Verification items for the finished model (mm, model axes). A direction names the side the tool comes from. Give positions to 0.01 mm unless a question says otherwise; leave off trailing zeros. Write each loop counter-clockwise with the first axis right and the second up, starting at its lowest first coordinate (ties: lowest second). Pieces come first, ordered by that corner, then holes. Notation, with made-up numbers: M 63.25,9.5 L 72.25,9.5 A30 ccw 72.25,40.5 Z; hole C 59,-30.5 d1. An arc over 180 degrees is marked long. Write item = value, one per line.
from build123d import *

# Parameters (mm, degrees)
F0_W     = 76.2
F0_H     = 76.2
F1_DEPTH = 25.4
F2_W     = 12.7
F2_H     = 76.2
F6_DEPTH = 25.4
F4_W     = 76.2
F4_H     = 12.7
F7_DEPTH = 25.4
F5_W     = 76.2
F5_H     = 12.7
F8_DEPTH = 25.4
F3_W     = 12.7
F3_H     = 76.2
F9_DEPTH = 25.4


with BuildPart() as f1:
    # F0 (on Top) → F1 (new body)
    with BuildSketch(Plane.XY):
        with Locations((0.213519, -0.247781)):
            Rectangle(F0_W, F0_H)
    extrude(amount=F1_DEPTH)

    # F2 (on Top) → F6 (join)
    with BuildSketch(Plane.XY):
        with Locations((0.173656, 75.769984)):
            Rectangle(F2_W, F2_H)
    extrude(amount=F6_DEPTH)

    # F4 (on Top) → F7 (join)
    with BuildSketch(Plane.XY):
        with Locations((-75.986146, -0.193442)):
            Rectangle(F4_W, F4_H)
    extrude(amount=F7_DEPTH)

    # F5 (on Top) → F8 (join)
    with BuildSketch(Plane.XY):
        with Locations((76.36796, -0.207913)):
            Rectangle(F5_W, F5_H)
    extrude(amount=F8_DEPTH)

    # F3 (on Top) → F9 (join)
    with BuildSketch(Plane.XY):
        with Locations((0.085362, -76.094228)):
            Rectangle(F3_W, F3_H)
    extrude(amount=F9_DEPTH)


solid = f1.part
1) Material ranges on probe 1 along Y at (x, z) = (-19.5, 1.5); probe 2 along X at (y, z) = (-29.5, 14); probe 3 along Y at (x, z) = (41, 16), recorded low to high. Write a range as from..to.
From the geometry:
probe_1 = -38.35..37.85
probe_2 = -37.89..38.31
probe_3 = -6.56..6.14
2) Cross-section at B-B on y = 53. Record the boundary of the cut face in (x, z), plus the area to 3 significant figures.
From the geometry:
outline = M -6.18,0 L 6.52,0 L 6.52,25.4 L -6.18,25.4 Z
area = 323 mm^2
3) Cross-section at A-A on z = 14. Record the boundary of the cut face in (x, y), plus the area to 3 significant figures.
From the geometry:
outline = M -114.09,-6.54 L -37.89,-6.54 L -37.89,-38.35 L -6.26,-38.35 L -6.26,-114.19 L 6.44,-114.19 L 6.44,-38.35 L 38.31,-38.35 L 38.31,-6.56 L 114.47,-6.56 L 114.47,6.14 L 38.31,6.14 L 38.31,37.85 L 6.52,37.85 L 6.52,113.87 L -6.18,113.87 L -6.18,37.85 L -37.89,37.85 L -37.89,6.16 L -114.09,6.16 Z
area = 9,670 mm^2
4) Depth check by flat-ended pin: P1, Ø7.5, axis at x = 23, z = 9, coming from the -Y side; P2, Ø12.5, axis at x = -58, z = 11, coming from the -Y side; P3, Ø12.5, axis at x = 77.5, z = 16, coming from the -Y side. Enter the tip coordinate at first touch or a pass-through.
From the geometry:
P1 = -38.35
P2 = -6.54
P3 = -6.56
5) Cross-section at C-C on x = -17. Record the boundary of the cut face in (y, z).
From the geometry:
outline = M -38.35,0 L 37.85,0 L 37.85,25.4 L -38.35,25.4 Z
6) Tool access check on faces 1 (the flat face through (6.435, -77, 13)), 2 (the flat face through (38.314, 22, 13)), 3 (the flat face through (0, -114.194, 13)), 4 (the flat face through (-37.886, 22, 13)), 5 (the flat face through (-22, -38.348, 13)). Record the directions out of +Z, -Z, +X, -X, +Y, -Y that give a thin tool (end or side, any length) a straight path to the whole face; none if there is none.
From the geometry:
face_1 = +Z, -Z, +X, -Y
face_2 = +Z, -Z, +X, +Y
face_3 = +Z, -Z, +X, -X, -Y
face_4 = +Z, -Z, -X, +Y
face_5 = +Z, -Z, -X, -Y
